Geometry check sheet. Reference: the model listing, model coordinates, mm. Round coordinates to 2 decimals unless told otherwise and drop trailing zeros. Loops run counter-clockwise (first coordinate to the right, second up) from the corner with the lowest first, then second, coordinate; pieces in that order, holes last. Notation, with made-up numbers: M 1.25,77.25 L 43.25,77.25 A23 cw 43.25,103.25 Z; hole C 2,12 d2. An arc over 180 degrees is marked long. Write item = value, one per line.
from build123d import *

# Parameters (mm, degrees)
F1_DEPTH = 18.288
F2_W     = 18.288
F2_H     = 76.2
F3_DEPTH = 25.4


with BuildPart() as f1:
    # F0 (on Top) → F1 (new body)
    with BuildSketch(Plane.XY):
        Polygon((-1067.61384, 176.902703), (-1067.61384, -32.647297), (-858.06384, -32.647297), (-858.06384, -50.935297), (-781.86384, -50.935297), (-781.86384, -32.647297), (-572.31384, -32.647297), (-572.31384, -50.935297), (-496.11384, -50.935297), (-496.11384, -32.647297), (-286.56384, -32.647297), (-286.56384, -50.935297), (-210.36384, -50.935297), (-210.36384, -32.647297), (-0.81384, -32.647297), (-458.01384, 176.902703), align=None)
    extrude(amount=F1_DEPTH)

    # F2 (on Top) → F3 (cut)
    with BuildSketch(Plane.XY):
        with Locations((-1032.45726, 73.806196)):
            Rectangle(F2_W, F2_H)
    extrude(amount=F3_DEPTH, mode=Mode.SUBTRACT)


solid = f1.part
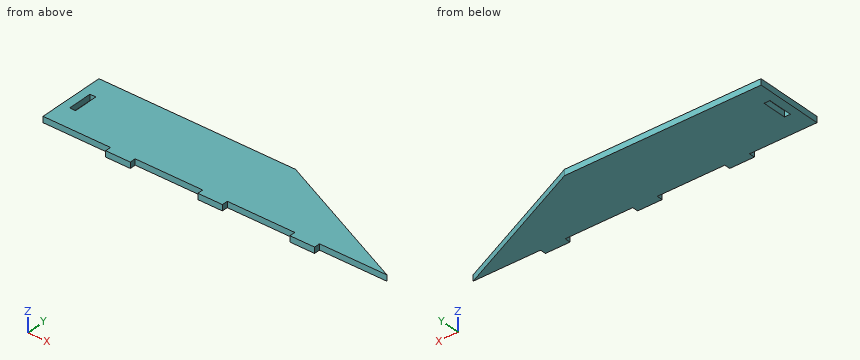
(1) Material ranges on line 1 along Y through (x, z) = (-466.5, 5); line 2 along X through (y, z) = (48, 11.5); line 3 along X through (y, z) = (83.5, 7), recorded low to high. Write a range as from..to.
Result set:
line_1 = -32.65..176.9
line_2 = -1067.61..-1041.6, -1023.31..-176.77
line_3 = -1067.61..-1041.6, -1023.31..-254.23
(2) Depth check by flat-ended pin: pin 1 Ø5.5 at (y, z) = (-39.5, 9.5) entering from +X; pin 2 Ø5 at (x, z) = (-367.5, 9.5) entering from -Y; pin 3 Ø1.5 at (x, z) = (-342.5, 14.5) entering from +Y. Enter the tip coordinate at first touch or a pass-through.
Result set:
pin_1 = -210.36
pin_2 = -32.65
pin_3 = 124.3
(3) Sectioned sample at A-A on z = 14. Record the cut outline in (x, y), then the cut area to 3 significant figures.
Result set:
outline = M -1067.61,-32.65 L -858.06,-32.65 L -858.06,-50.94 L -781.86,-50.94 L -781.86,-32.65 L -572.31,-32.65 L -572.31,-50.94 L -496.11,-50.94 L -496.11,-32.65 L -286.56,-32.65 L -286.56,-50.94 L -210.36,-50.94 L -210.36,-32.65 L -0.81,-32.65 L -458.01,176.9 L -1067.61,176.9 Z; hole M -1041.6,35.71 L -1023.31,35.71 L -1023.31,111.91 L -1041.6,111.91 Z
area = 178,000 mm2
(4) Sectioned sample at C-C on x = -643. Record the cut outline in (y, z).
Result set:
outline = M -32.65,0 L 176.9,0 L 176.9,18.29 L -32.65,18.29 Z
(5) Sectioned sample at D-D on y = 22. Record the cut outline in (x, z).
Result set:
outline = M -1067.61,0 L -120.04,0 L -120.04,18.29 L -1067.61,18.29 Z
(6) Sectioned sample at B-B on y = 84. Record the cut outline in (x, z), then the cut area to 3 significant figures.
Result set:
outline = M -1067.61,0 L -1041.6,0 L -1041.6,18.29 L -1067.61,18.29 Z; M -1023.31,0 L -255.32,0 L -255.32,18.29 L -1023.31,18.29 Z
area = 14,500 mm2
